Geometry: final body of the model. Coordinates: model frame, mm. A direction names the side the tool comes from. Round coordinates to 2 decimals unless told otherwise and drop trailing zeros. Loops run counter-clockwise (first coordinate to the right, second up) from the corner with the lowest first, then second, coordinate; pieces in that order, holes last. Notation, with made-up numbers: M 10.25,-10 L 29.25,-10 A19 ccw 29.25,6 Z; hole C 47.5,22 d6. An arc over 180 degrees is marked long. Write each question's results on one line, items separated by ' | '.
```python
from build123d import *

# Parameters (mm, degrees)
F0_W     = 200
F0_H     = 200
F1_DEPTH = 25
F2_W     = 169.5
F2_H     = 169.5
F3_DEPTH = 25
F3_TAPER = 25
F4_W     = 22
F4_H     = 30
F5_DEPTH = 5


with BuildPart() as f1:
    # F0 (on Right) → F1 (new body)
    with BuildSketch(Plane.YZ):
        with Locations((100, 100)):
            Rectangle(F0_W, F0_H)
    extrude(amount=F1_DEPTH)

    # F2 (on face) → F3 (join)
    with BuildSketch(Plane(origin=(0, 0, 0), x_dir=(0, -1, 0), z_dir=(-1, 0, 0))):
        with Locations((-100, 100)):
            Rectangle(F2_W, F2_H)
    extrude(amount=F3_DEPTH, taper=F3_TAPER)

    # F4 (on face) → F5 (cut)
    with BuildSketch(Plane(origin=(0, 0, 0), x_dir=(1, 0, 0), z_dir=(0, 0, -1))):
        with Locations((11, -165)):
            Rectangle(F4_W, F4_H)
        with Locations((11, -35)):
            Rectangle(F4_W, F4_H)
    extrude(amount=-F5_DEPTH, mode=Mode.SUBTRACT)


solid = f1.part
```
1. Pin query (flat end, axial travel): P1, Ø1.5, axis at x = -13.5, z = 113, coming from the +Y side; P2, Ø24, axis at x = 7, y = 36, coming from the -Z side; P3, Ø2, axis at x = -16, z = 161.5, coming from the -Y side. Return the tip coordinate at first contact, or that it passes through.
Answer key:
P1: stops at y = 178.8 | P2: stops at z = 5 | P3: stops at y = 22.24
2. Section A-A (z = 187.5). Output: boundary loops of the cut face in (x, y).
Answer key:
outline: M 0,0 L 25,0 L 25,200 L 0,200 Z
3. Ray query, probe 1 along X at (y, z) = (189, 43); probe 2 along Z at (x, y) = (15.5, 39.5); probe 3 along X at (y, z) = (128, 174). Return the intervals inside material, ascending.
Answer key:
probe 1: x = 0 to 25 | probe 2: z = 5 to 200 | probe 3: x = -23.05 to 25
4. Draft query along Y for faces 1 (the face through (11, 165, 5)), 2 (the face through (12, 200, 99)), 3 (the face through (25, 99, 101)). Return one class per face: pulls with the +Y half, pulls with the -Y half, needs draft (parallel to the pull), parting line crosses it, or undercut.
Answer key:
face 1: undercut | face 2: pulls with the +Y half | face 3: needs draft
5. Access query for faces 4 (the face through (11, 180, 2)), 5 (the face through (0, 187, 101)), 6 (the face through (-25, 102, 100)). Directions: +Z, -Z, +X, -X, +Y, -Y. A direction counts if a zero-diameter tool reaches every point of the face in a straight line with its end or side. Return the directions, or none.
Answer key:
face 4: -Z, -X | face 5: -X | face 6: +Z, -Z, -X, +Y, -Y
